Autodesk Inventor part; units mm, degrees
ref_plane "YZ Plane" through (0, 0, 0) normal (1, 0, 0) x (0, 1, 0)
ref_plane "XZ Plane" through (0, 0, 0) normal (0, 1, 0) x (-1, 0, 0)
ref_plane "XY Plane" through (0, 0, 0) normal (0, 0, 1) x (1, 0, 0)
sketch "Esboço1" plane through (0, 0, 0) normal (0, 1, 0) x (-1, 0, 0)
  line L0 (-83.8742, 0) -> (0, 0)
  line L1 (0, 0) -> (0, 3)
  line L2 (0, 3) -> (-83.8742, 3)
  line L3 (-83.8742, 3) -> (-83.8742, 0)
  dimension "d0" = 3
extrude "Extrusão1" add sketch "Esboço1" along normal blind 138.2
ref_plane "Plano de trabalho1" through (83.8742, 109.1, 0) normal (-0.1736, 0, 0.9848) x (0, -1, 0)
sketch "Esboço2" plane through (83.8742, 109.1, 0) normal (-0.1736, 0, 0.9848) x (0, -1, 0)
  line L0 (0.8787, 5.1213) -> (-31.2213, -26.9787)
  line L1 (79.1213, 5.1213) -> (111.2213, -26.9787)
  line L2 (120.2426, -26.2032) -> (-42, -26.2032)
  line L3 (-42, -26.2032) -> (-42, 2.623)
  line L4 (-42, 2.623) -> (120.2426, 2.623)
  line L5 (120.2426, 2.623) -> (120.2426, -26.2032)
  point P0 (109.1, -82.6)
  point P1 (-30.4458, -26.2032)
  point P2 (-1.6196, 2.623)
  point P3 (81.6196, 2.623)
  point P4 (110.4458, -26.2032)
extrude "Extrusão2" cut sketch "Esboço2" along normal blind 13.7 contours L0 L2 L3 L4 | L4 L5 L2 L1
properties part number "tampa"
Read the model definition and answer for the solid it produces. Units are mm, in the model's axes. Coordinates: 2 decimals unless noted, no trailing zeros. Write each loop counter-clockwise with the first axis right and the second up, starting at its lowest first coordinate (ties: lowest second). Pieces come first, ordered by that corner, then holes. Notation, with made-up numbers: (47, 57) -> (54, 57) arc R14 cw to (54, 75) -> close; hole circle Ø6 at (0, 80.5). An arc over 180 degrees is marked (long way). Return JSON: item names as keys, results as strings.
(1) Consider line 1 along X through (y, z) = (119, 0.3); line 2 along X through (y, z) = (121, 1.4); line 3 along Y through (x, z) = (79, 2.1). Determine where each line is inside the solid, lowest interval first. Write a range as from..to.
Answers below:
{"line 1": "0..78.08", "line 2": "0..75.85", "line 3": "20.42..117.78"}
(2) The part is cut by section A-A on z = 1.3. Give the vertices of the cut face in (x, y).
Answers below:
{"outline": "(0, 0) -> (58.4, 0) -> (83.87, 25.08) -> (83.87, 113.12) -> (58.4, 138.2) -> (0, 138.2) -> close"}
(3) The part is cut by section C-C on x = 60. Give the vertices of the cut face in (y, z).
Answers below:
{"outline": "(1.35, 0) -> (136.85, 0) -> (136.33, 3) -> (1.87, 3) -> close"}
(4) The part is cut by section B-B on y = 8. Give the vertices of the cut face in (x, z), then the cut area to 3 significant figures.
Answers below:
{"outline": "(0, 0) -> (66.76, 0) -> (66.23, 3) -> (0, 3) -> close", "area": "199 mm^2"}
